Source: CAD feature listing. Evaluate the final solid. Frame: model axes, mm. A direction names the side the tool comes from. Round coordinates to 2 decimals unless told otherwise and drop trailing zeros. Write each loop counter-clockwise with the first axis right and the second up, starting at its lowest first coordinate (ties: lowest second). Pieces come first, ordered by that corner, then holes. Notation, with made-up numbers: M 10,5 L 34,5 A32 ccw 34,37 Z; hole C 10.5,-40 d9. An arc over 180 degrees is marked long. Answer in a Markdown table with one row per item.
from build123d import *

# Parameters (mm, degrees)
F1_DEPTH = 0.9
F0_W     = 20
F0_H     = 6
F2_DEPTH = 2.5


with BuildPart() as f1:
    # F0 (on Top) → F1 (new body)
    with BuildSketch(Plane.XY):
        Polygon((-0.1961524227, -11.6602540378), (-10.1961524227, 5.6602540378), (-15.3923048454, 2.6602540378), (-5.3923048454, -14.6602540378), align=None)
    extrude(amount=F1_DEPTH)



with BuildPart() as f1b:
    # F0 (on Top) → F1, piece 2 (new body)
    with BuildSketch(Plane.XY):
        with Locations((0, 9)):
            Rectangle(F0_W, F0_H)
    extrude(amount=F1_DEPTH)


with BuildPart() as f1c:
    # F0 (on Top) → F1, piece 3 (new body)
    with BuildSketch(Plane.XY):
        Polygon((15.3923048454, 2.6602540378), (10.1961524227, 5.6602540378), (0.1961524227, -11.6602540378), (5.3923048454, -14.6602540378), align=None)
    extrude(amount=F1_DEPTH)


with BuildPart() as f1_1:
    add(f1.part)

    add(f1b.part)  # F2 merges F1b

    add(f1c.part)  # F2 merges F1c
    # F0 (on Top) → F2 (join)
    with BuildSketch(Plane.XY):
        Polygon((10, 6), (-10, 6), (-10.1961524227, 5.6602540378), (-0.1961524227, -11.6602540378), (0.1961524227, -11.6602540378), (10.1961524227, 5.6602540378), align=None)
        Polygon((6.9282032303, 4), (0, -8), (-6.9282032303, 4), align=None, mode=Mode.SUBTRACT)
    extrude(amount=F2_DEPTH)


solid = f1_1.part
Q1. Access query for faces 1 (the flat face through (0, 4, 1)), 2 (the flat face through (-8, -4, 0.9)), 3 (the flat face through (0, 9, 0.9)), 4 (the flat face through (-2.83, -13.18, 0.44)), 5 (the flat face through (10, 9, 0.4)). Directions: +Z, -Z, +X, -X, +Y, -Y. A direction counts if a zero-diameter tool reaches every point of the face in a straight line with its end or side. Return the directions, or none.
Solutions:
| item | result |
|---|---|
| face 1 | +Z, -Z |
| face 2 | +Z, -X, -Y |
| face 3 | +Z, +X, -X, +Y |
| face 4 | +Z, -Z, -Y |
| face 5 | +Z, -Z, +X, +Y |
Q2. Material intervals for probe 1 along Z at (x, y) = (-4.5, 9.25); probe 2 along Y at (x, z) = (-3.5, 0.8); probe 3 along X at (y, z) = (3.75, 0.3), sorted ascending.
Solutions:
| item | result |
|---|---|
| probe 1 | z = 0 to 0.9 |
| probe 2 | y = -13.57 to -1.94, 4 to 12 |
| probe 3 | x = -13.5 to -6.78, 6.78 to 13.5 |
Q3. Section D-D (y = 10). Return loops of the section in (x, z).
Solutions:
| item | result |
|---|---|
| outline | M -10,0 L 10,0 L 10,0.9 L -10,0.9 Z |
Q4. Pull-direction query (Y, two-part tool) for faces 6 (the flat face through (-3.42, -2.08, 1.23)), 7 (the flat face through (5.126, -3.121, 1.689)), 8 (the flat face through (-0.1, 12, 0.4)), 9 (the flat face through (-10, 9, 0.4)); classes: pulls with the +Y half, pulls with the -Y half, needs draft (parallel to the pull), parting line crosses it, or undercut.
Solutions:
| item | result |
|---|---|
| face 6 | undercut |
| face 7 | pulls with the -Y half |
| face 8 | pulls with the +Y half |
| face 9 | needs draft |
Q5. Section B-B (y = -12). Return loops of the section in (x, z), and give its area (3 significant figures).
Solutions:
| item | result |
|---|---|
| outline | M -6.93,0 L -0.78,0 L -0.78,0.9 L -6.93,0.9 Z; M 0.78,0 L 6.93,0 L 6.93,0.9 L 0.78,0.9 Z |
| area | 11.1 mm2 |
Q6. Section C-C (x = -1). Return loops of the section in (y, z).
Solutions:
| item | result |
|---|---|
| outline | M -12.12,0 L -6.27,0 L -6.27,2.5 L -10.27,2.5 L -10.27,0.9 L -12.12,0.9 Z; M 4,0 L 12,0 L 12,0.9 L 6,0.9 L 6,2.5 L 4,2.5 Z |
Q7. Contact query for flat-ended pins moving along their axis: pin 1 Ø1.5 at (y, z) = (-2, 2) entering from +X; pin 2 Ø12 at (x, y) = (-7, -7) entering from +Z; pin 3 Ø0.7 at (y, z) = (10, 0.5) entering from -X; pin 4 Ø1.5 at (x, y) = (-11, -5.5) entering from +Z. Output: stop coordinate, or through.
Solutions:
| item | result |
|---|---|
| pin 1 | stops at x = 6.21 |
| pin 2 | stops at z = 2.5 |
| pin 3 | stops at x = -10 |
| pin 4 | stops at z = 0.9 |
Q8. Section A-A (z = 1.75). Return loops of the section in (x, y).
Solutions:
| item | result |
|---|---|
| outline | M -10.2,5.66 L -0.2,-11.66 L 0.2,-11.66 L 10.2,5.66 L 10,6 L -10,6 Z; hole M -6.93,4 L 0,-8 L 6.93,4 Z |
